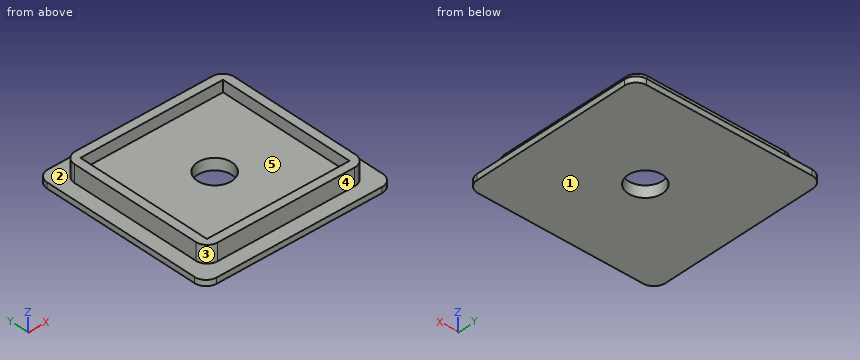
from build123d import *

# Parameters (mm, degrees)
F0_W     = 25
F0_H     = 24
F0_R     = 3
F1_DEPTH = 2
F2_DEPTH = 4
F3_DEPTH = 1


with BuildPart() as f1:
    # F0 (on Top) → F1 (new body)
    with BuildSketch(Plane.XY):
        with Locations((0, -0.065946)):
            Rectangle(F0_W, F0_H)
        Circle(F0_R, mode=Mode.SUBTRACT)
    extrude(amount=F1_DEPTH)

    # F0 (on Top) → F2 (join)
    with BuildSketch(Plane.XY):
        with BuildLine():
            Line((12, 13.434054), (-12, 13.434054))
            ThreePointArc((-12, 13.434054), (-13.414214, 12.848268), (-14, 11.434054))
            Line((-14, 11.434054), (-14, -11.565946))
            ThreePointArc((-14, -11.565946), (-13.414214, -12.98016), (-12, -13.565946))
            Line((-12, -13.565946), (12, -13.565946))
            ThreePointArc((12, -13.565946), (13.414214, -12.98016), (14, -11.565946))
            Line((14, -11.565946), (14, 11.434054))
            ThreePointArc((14, 11.434054), (13.414214, 12.848268), (12, 13.434054))
        make_face()
        with Locations((0, -0.065946)):
            Rectangle(F0_W, F0_H, mode=Mode.SUBTRACT)
    extrude(amount=F2_DEPTH)

    # F0 (on Top) → F3 (join)
    with BuildSketch(Plane.XY):
        with BuildLine():
            Line((14.5, 15.934054), (-14.5, 15.934054))
            ThreePointArc((-14.5, 15.934054), (-15.914214, 15.348268), (-16.5, 13.934054))
            Line((-16.5, 13.934054), (-16.5, -14.065946))
            ThreePointArc((-16.5, -14.065946), (-15.914214, -15.48016), (-14.5, -16.065946))
            Line((-14.5, -16.065946), (14.5, -16.065946))
            ThreePointArc((14.5, -16.065946), (15.914214, -15.48016), (16.5, -14.065946))
            Line((16.5, -14.065946), (16.5, 13.934054))
            ThreePointArc((16.5, 13.934054), (15.914214, 15.348268), (14.5, 15.934054))
        make_face()
        with BuildLine():
            ThreePointArc((-14, 11.434054), (-13.414214, 12.848268), (-12, 13.434054))
            Line((-12, 13.434054), (12, 13.434054))
            ThreePointArc((12, 13.434054), (13.414214, 12.848268), (14, 11.434054))
            Line((14, 11.434054), (14, -11.565946))
            ThreePointArc((14, -11.565946), (13.414214, -12.98016), (12, -13.565946))
            Line((12, -13.565946), (-12, -13.565946))
            ThreePointArc((-12, -13.565946), (-13.414214, -12.98016), (-14, -11.565946))
            Line((-14, -11.565946), (-14, 11.434054))
        make_face(mode=Mode.SUBTRACT)
    extrude(amount=F3_DEPTH)


solid = f1.part
Can you work these out from the model? Positions are in its coordinate system, mm. Face numbers are marked on the shaded views. A direction names the side the tool comes from. Coordinates: 2 decimals unless noted, no trailing zeros. Order: outer loops, then holes, each group sorted by start corner. A loop starts at its lowest first (then second) coordinate and runs counter-clockwise, first axis right, second up. Notation, with made-up numbers: (-10, 35) - (0, 35) arc R17 cw to (0, 46) - close; hole circle Ø5 at (5, 79.25). An arc over 180 degrees is marked (long way). Answer as a JSON object with one key per item and string values. Group by question number.
Q1. I need wall thicknesses on line 1 (Y direction, x = 0, z = 0.85); line 2 (Y direction, x = 6, z = 2.05); line 3 (X direction, y = 7.5, z = 3.8). Which ranges of each line are inside material? Lowest first, please. Write a range as from..to.
Q2. Imagine slicing it at B-B (z = 2.6). Please give me the cut outline in (x, y).
Q3. Imagine slicing it at C-C (y = 0). Please give me the cut outline in (x, z).
Q4. Imagine slicing it at D-D (x = -8). Please give me the cut outline in (y, z).
Q5. Imagine slicing it at A-A (x = 0). Please give me the cut outline in (y, z), and give its area (3 significant figures).
Q6. We'd pull the mould along X, two halves only. Please class the marked faces 3, 4 and 5: +X half, -X half, draft (parallel to the pull), parting line (faces both ways), or undercut.
Q7. Will these pins go through, and if not, where does the flat tip stop? P1, Ø1, axis at y = -3.5, z = 2.5, coming from the -X side; P2, Ø1, axis at x = 6.5, y = 8.5, coming from the -Z side; P3, Ø7, axis at x = 0, y = 0, coming from the +Z side; P4, Ø1.6, axis at x = 3.5, z = 3, coming from the -Y side.
Q8. On a 3-axis mill with a long thin cutter (end or side, diameter ignored), from which of +Z, -Z, +X, -X, +Y, -Y can I reach the whole of each face in a straight line? I mean the marked faces 1 and 2. Say none if no direction works.
Determined:
{
 "1": {"line 1": "y = -16.07..-3, 3..15.93", "line 2": "y = -13.57..-12.07, 11.93..13.43", "line 3": "x = -14..-12.5, 12.5..14"},
 "2": {"outline": "(-14, -11.57) arc R2 ccw to (-12, -13.57) - (12, -13.57) arc R2 ccw to (14, -11.57) - (14, 11.43) arc R2 ccw to (12, 13.43) - (-12, 13.43) arc R2 ccw to (-14, 11.43) - close; hole (-12.5, -12.07) - (12.5, -12.07) - (12.5, 11.93) - (-12.5, 11.93) - close"},
 "3": {"outline": "(-16.5, 0) - (-3, 0) - (-3, 2) - (-12.5, 2) - (-12.5, 4) - (-14, 4) - (-14, 1) - (-16.5, 1) - close; (3, 0) - (16.5, 0) - (16.5, 1) - (14, 1) - (14, 4) - (12.5, 4) - (12.5, 2) - (3, 2) - close"},
 "4": {"outline": "(-16.07, 0) - (15.93, 0) - (15.93, 1) - (13.43, 1) - (13.43, 4) - (11.93, 4) - (11.93, 2) - (-12.07, 2) - (-12.07, 4) - (-13.57, 4) - (-13.57, 1) - (-16.07, 1) - close"},
 "5": {"outline": "(-16.07, 0) - (-3, 0) - (-3, 2) - (-12.07, 2) - (-12.07, 4) - (-13.57, 4) - (-13.57, 1) - (-16.07, 1) - close; (3, 0) - (15.93, 0) - (15.93, 1) - (13.43, 1) - (13.43, 4) - (11.93, 4) - (11.93, 2) - (3, 2) - close", "area": "53.0 mm2"},
 "6": {"face 3": "-X half", "face 4": "draft", "face 5": "undercut"},
 "7": {"P1": "stops at x = -14", "P2": "stops at z = 0", "P3": "stops at z = 2", "P4": "stops at y = -13.57"},
 "8": {"face 1": "-Z, +X, -X, +Y, -Y", "face 2": "+Z"}
}
